The drawing under review shows one solid part. Ordinate dimensions are in mm from its lowest x, y, z. Coordinates: 2 decimals unless noted, no trailing zeros. Order: outer loops, then holes, each group sorted by start corner. A loop starts at its lowest first (then second) coordinate and runs counter-clockwise, first axis right, second up. Notation, with made-up numbers: (-39.75, 26.5) - (17.25, 26.5) arc R4 ccw to (17.25, 31.5) - close; hole circle Ø5 at (72, -18). An arc over 180 degrees is marked (long way). Write each question's results on one line, items separated by ' | '. Start each with the question number.
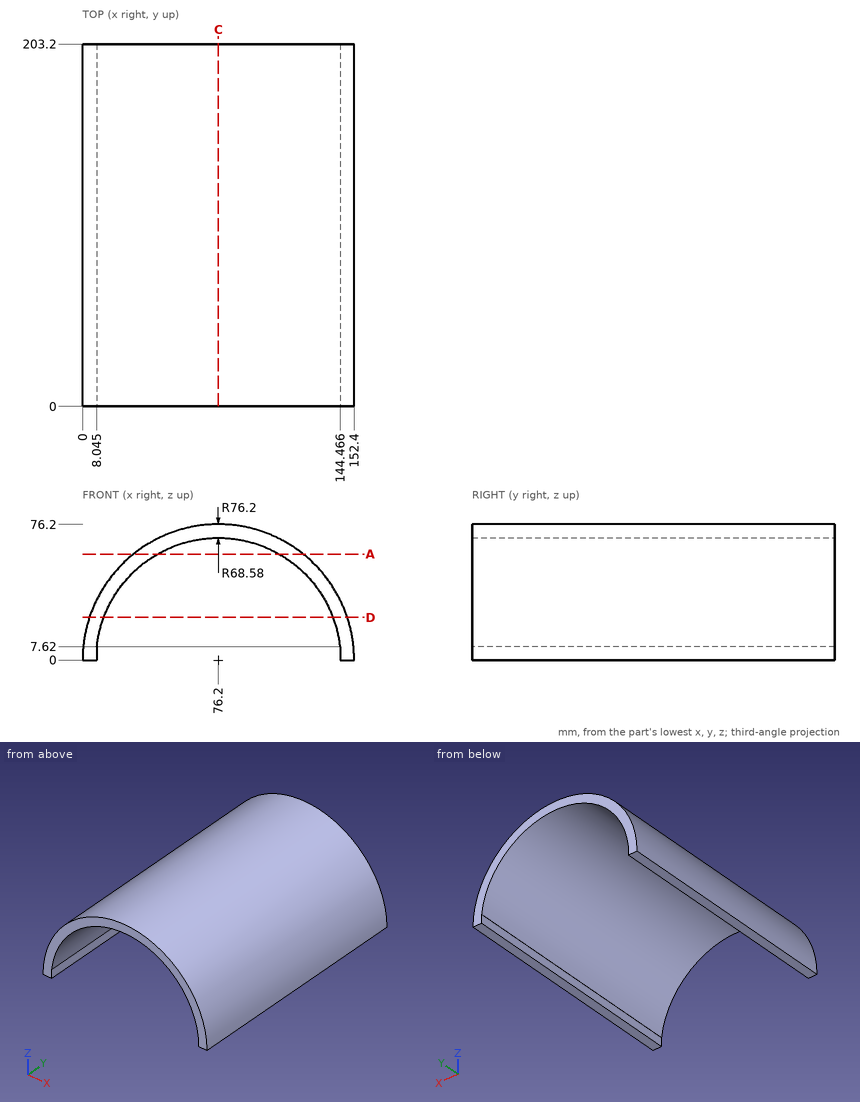
(1) To check wall thickness, follow line 1 along X through (y, z) = (76, 47); line 2 along X through (y, z) = (167, 44.5) (1 decimal); line 3 along Z through (x, y) = (124, 77) (1 decimal). State the ranges of each line that lie inside material, in increasing order. Write a range as [from, to].
(2) Take a section at C-C (x = 76.2). State the section outline as (y, z) points.
(3) Take a section at A-A (z = 59.5). State the section outline as (x, y) points (1 decimal), plus the area to 3 significant figures.
(4) Take a section at D-D (z = 24). State the section outline as (x, y) points.
(5) Clearance check with flat-ended pins moving along their axes: pin 1 (3 mm diameter, centred on x = 43, y = 166.5, fed in from -Z); pin 2 (3 mm diameter, centred on x = 102, y = 46.5, fed in from +Z); pin 3 (1.5 mm diameter, centred on y = 44.5, z = 40, fed in from -X). State where each tip first meets the part, or that it passes through.
Worked out:
1) line 1: [16.22, 26.26], [126.14, 136.18] | line 2: [14.3, 24], [128.4, 138.1] | line 3: [49.2, 59.3]
2) outline: (0, 68.58) - (203.2, 68.58) - (203.2, 76.2) - (0, 76.2) - close
3) outline: (28.6, 0) - (42.1, 0) - (42.1, 203.2) - (28.6, 203.2) - close; (110.3, 0) - (123.8, 0) - (123.8, 203.2) - (110.3, 203.2) - close | area: 5,490 mm^2
4) outline: (3.88, 0) - (11.96, 0) - (11.96, 203.2) - (3.88, 203.2) - close; (140.44, 0) - (148.52, 0) - (148.52, 203.2) - (140.44, 203.2) - close
5) pin 1: z = 59.15 | pin 2: z = 72.22 | pin 3: x = 10.89
